from build123d import *

# Parameters (mm, degrees)
SKETCH1_R           = 6
BOSS_EXTRUDE1_DEPTH = 33
SKETCH7_R           = 4.5
BOSS_EXTRUDE7_DEPTH = 2.54
SKETCH3_R           = 6
BOSS_EXTRUDE3_DEPTH = 5
SKETCH4_R           = 4.45
BOSS_EXTRUDE4_DEPTH = 2.54
CUT_EXTRUDE1_DEPTH  = 31.5


with BuildPart() as part:
    # Sketch1 → Boss-Extrude1 (new body)
    with BuildSketch(Plane.XY):
        Circle(SKETCH1_R)
    extrude(amount=BOSS_EXTRUDE1_DEPTH)

    # Sketch7 → Boss-Extrude7 (add)
    with BuildSketch(Plane.XY.offset(33)):
        Circle(SKETCH7_R)
    extrude(amount=BOSS_EXTRUDE7_DEPTH)

    # Sketch3 → Boss-Extrude3 (add)
    with BuildSketch(Plane.XY.offset(35.54)):
        with Locations((0, 0.6604)):
            Circle(SKETCH3_R)
    extrude(amount=BOSS_EXTRUDE3_DEPTH)

    # Sketch4 → Boss-Extrude4 (add)
    with BuildSketch(Plane.XY.offset(40.54)):
        Circle(SKETCH4_R)
    extrude(amount=BOSS_EXTRUDE4_DEPTH)

    # Sketch5 → Cut-Extrude1 (cut)
    with BuildSketch(Plane(origin=(0, 0, 0), x_dir=(-1, 0, 0), z_dir=(0, 0, -1))):
        with BuildLine():
            Line((-1.075, 5.09246155), (-1.075, 3.98246155))
            ThreePointArc((-1.075, 3.98246155), (0, 4.125), (1.075, 3.98246155))
            Line((1.075, 3.98246155), (1.075, 5.09246155))
            Line((1.075, 5.09246155), (-1.075, 5.09246155))
        make_face()
        with BuildLine():
            ThreePointArc((1.075, 3.98246155), (0, 4.125), (-1.075, 3.98246155))
            Line((-1.075, 3.98246155), (1.075, 3.98246155))
        make_face()
        with BuildLine():
            Line((1.075, 3.98246155), (-1.075, 3.98246155))
            ThreePointArc((-1.075, 3.98246155), (-2.50811184, -3.274904579), (4.125, 0))
            ThreePointArc((4.125, 0), (3.274904579, 2.50811184), (1.075, 3.98246155))
        make_face()
    extrude(amount=-CUT_EXTRUDE1_DEPTH, mode=Mode.SUBTRACT)


solid = part.part
Build history of the part. All positions in model axes, mm. A direction names the side the tool comes from. Give positions to 0.01 mm unless a question says otherwise; leave off trailing zeros. Write each loop counter-clockwise with the first axis right and the second up, starting at its lowest first coordinate (ties: lowest second). Pieces come first, ordered by that corner, then holes. Notation, with made-up numbers: (39, 28) - (80, 28) arc R23 cw to (80, 43) - close; hole circle Ø3 at (89, -39.5). An arc over 180 degrees is marked (long way). Use one line per item in the form item = value. Start each with the question number.
1. Drop flat-ended pins along their axis: pin 1 Ø1.5 at (x, z) = (-1, 18) entering from -Y; pin 2 Ø1 at (y, z) = (-3, 26) entering from +X; pin 3 Ø6 at (x, y) = (2, 3.5) entering from -Z; pin 4 Ø2 at (y, z) = (2, 32) entering from -X. Give the stop position or say it passes through.
2. Band-saw the part on A-A on z = 22.5. Write the cut outline in (x, y) (3 decimals).
3. 3-axis set-ups, long thin cutter, end or side, ignore diameter. For faces 1 (the face through (1.075, 4.5, 15.5)), 2 (the face through (-1.4, 4.5, 33)), 3 (the face through (-5.994, 0.924, 38.005)): which of +Z, -Z, +X, -X, +Y, -Y reach the whole face in a straight line?
4. Band-saw the part on B-B on x = 0. Write the cut outline in (y, z) (3 decimals).
5. Two-plate mould, pull along X, no slides. Class faces 4 (the face through (-0.965, -4.344, 41.792)), 5 (the face through (0, 5, 40.54)), 6 (the face through (0, 5.092, 16)): released by +X, released by -X, zero draft, split by the parting line, or undercut.
6. Probe line 1 (Y direction, x = 0, z = 18) (3 decimals); line 2 (Z direction, x = -1.5, y = 4.5); line 3 (Z direction, x = 1.5, y = 3.75). List the from-to ranges inside material, lowest first. Write a range as [from, to].
7. Band-saw the part on C-C on y = -3.25. Write the cut outline in (x, z), plus the area to 3 significant figures.
Conclusion:
q1.pin_1 = -5.99
q1.pin_2 = 5.45
q1.pin_3 = 0
q1.pin_4 = -5.92
q2.outline = circle Ø12 at (0, 0); hole (-1.075, 3.982) arc R4.125 ccw (long way) to (1.075, 3.982) - (1.075, 5.092) - (-1.075, 5.092) - close
q3.face_1 = -Z
q3.face_2 = none
q3.face_3 = +Z
q4.outline = (-6, 0) - (-4.125, 0) - (-4.125, 31.5) - (5.092, 31.5) - (5.092, 0) - (6, 0) - (6, 33) - (4.5, 33) - (4.5, 35.54) - (6.66, 35.54) - (6.66, 40.54) - (4.45, 40.54) - (4.45, 43.08) - (-4.45, 43.08) - (-4.45, 40.54) - (-5.34, 40.54) - (-5.34, 35.54) - (-4.5, 35.54) - (-4.5, 33) - (-6, 33) - close
q5.face_4 = split by the parting line
q5.face_5 = zero draft
q5.face_6 = undercut
q6.line_1 = [-6, -4.125], [5.092, 6]
q6.line_2 = [0, 33], [35.54, 40.54]
q6.line_3 = [31.5, 43.08]
q7.outline = (-5.04, 0) - (-2.54, 0) - (-2.54, 31.5) - (2.54, 31.5) - (2.54, 0) - (5.04, 0) - (5.04, 33) - (3.11, 33) - (3.11, 35.54) - (4.55, 35.54) - (4.55, 40.54) - (3.04, 40.54) - (3.04, 43.08) - (-3.04, 43.08) - (-3.04, 40.54) - (-4.55, 40.54) - (-4.55, 35.54) - (-3.11, 35.54) - (-3.11, 33) - (-5.04, 33) - close
q7.area = 250 mm²
